Answer from the drawing. Dimensions are ordinates in mm from the lowest x, y and z of the part. A direction names the side the tool comes from. Coordinates: 2 decimals unless noted, no trailing zeros. Write each loop counter-clockwise with the first axis right and the second up, starting at its lowest first coordinate (ties: lowest second). Pieces come first, ordered by that corner, then holes.
(1) Determine the mould class of the marked faces 4, 5 and 6 for opening direction Z: pulls with the +Z half, pulls with the -Z half, needs draft (parallel to the pull), parting line crosses it, or undercut.
(2) Given pin 1 (4 mm diameter, centred on y = 18.5, z = 7.5, fed in from -X); pin 2 (8 mm diameter, centred on x = 6, z = 18, fed in from +Y); pin 3 (3 mm diameter, centred on x = 16, z = 16, fed in from +Y); pin 4 (13 mm diameter, centred on y = 33.5, z = 9, fed in from +X), each flat-ended and moving along its own axis, determine where each tip first touches the part or whether it passes through.
(3) The part is cut by section A-A, the plane z = 10.75. Determine the outline of the cut face in (x, y), and give its area (3 significant figures).
(4) Straight lines are drawn through the part: line 1 along Y through (x, z) = (10.25, 13); line 2 along X through (y, z) = (39, 24.5); line 3 along Y through (x, z) = (14.25, 16.5). For each, find the intervals that lie inside material, in ascending order.
(5) The part is cut by section B-B, the plane y = 30. Determine the outline of the cut face in (x, z), and give its area (3 significant figures).
(6) The part is cut by section D-D, the plane z = 13.75. Determine the outline of the cut face in (x, y).
(7) Which of the six approach directions +Z, -Z, +X, -X, +Y, -Y give full straight-line access (tool end or side, diameter ignored) to the marked faces 1, 2 and 3?
(8) The part is cut by section C-C, the plane x = 10.25. Determine the outline of the cut face in (y, z).
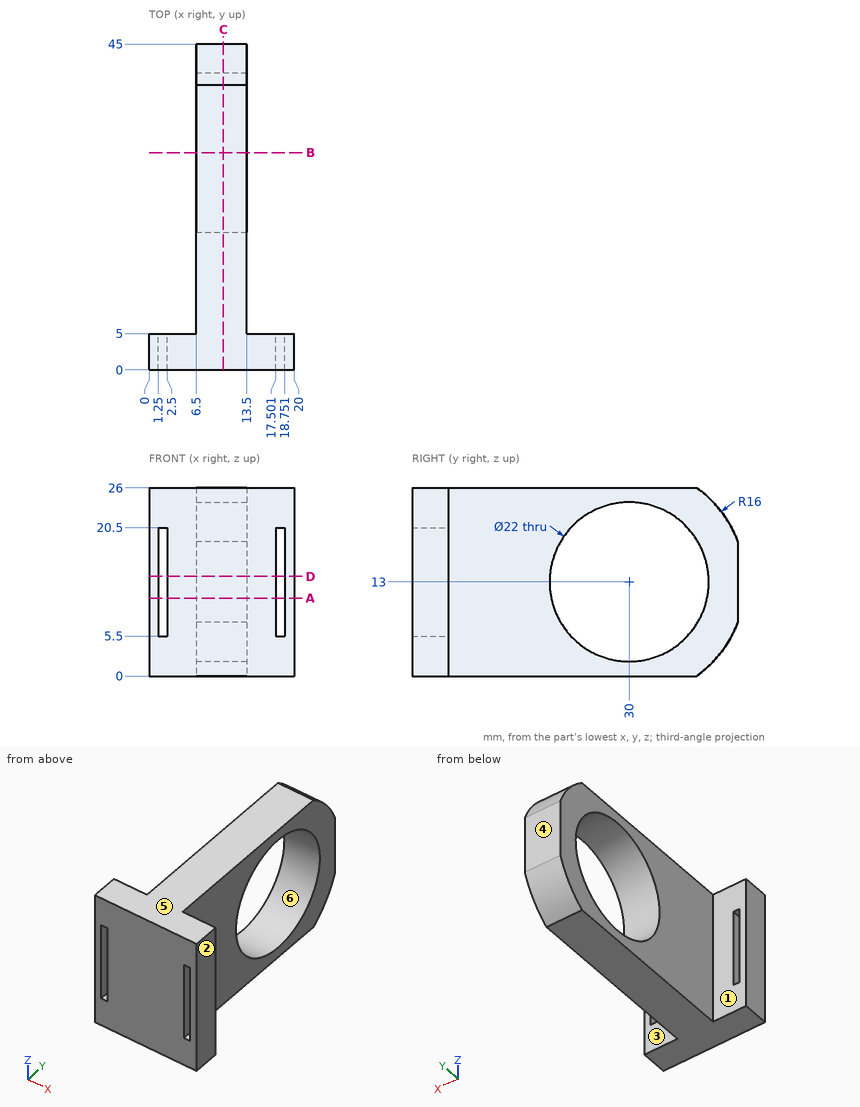
Computed:
1. face 4: needs draft
1. face 5: pulls with the +Z half
1. face 6: undercut
2. pin 1: stops at x = 6.5
2. pin 2: stops at y = 45
2. pin 3: stops at y = 5
2. pin 4: stops at x = 13.5
3. outline: (0, 0) - (1.25, 0) - (1.25, 5) - (0, 5) - close; (2.5, 0) - (17.5, 0) - (17.5, 5) - (13.5, 5) - (13.5, 19.23) - (6.5, 19.23) - (6.5, 5) - (2.5, 5) - close; (6.5, 40.77) - (13.5, 40.77) - (13.5, 45) - (6.5, 45) - close; (18.75, 0) - (20, 0) - (20, 5) - (18.75, 5) - close
3. area: 217 mm2
4. line 1: y = 0 to 19, 41 to 45
4. line 2: x = 6.5 to 13.5
4. line 3: y = 0 to 5
5. outline: (6.5, 0) - (13.5, 0) - (13.5, 2) - (6.5, 2) - close; (6.5, 24) - (13.5, 24) - (13.5, 26) - (6.5, 26) - close
5. area: 28.0 mm2
6. outline: (0, 0) - (1.25, 0) - (1.25, 5) - (0, 5) - close; (2.5, 0) - (17.5, 0) - (17.5, 5) - (13.5, 5) - (13.5, 19.03) - (6.5, 19.03) - (6.5, 5) - (2.5, 5) - close; (6.5, 40.97) - (13.5, 40.97) - (13.5, 45) - (6.5, 45) - close; (18.75, 0) - (20, 0) - (20, 5) - (18.75, 5) - close
7. face 1: +Z, -Z, -X, +Y
7. face 2: +Z, -Z, +X, +Y, -Y
7. face 3: +Z, -Z, +X, +Y
8. outline: (0, 0) - (39.33, 0) arc R16 ccw to (45, 7.43) - (45, 18.57) arc R16 ccw to (39.33, 26) - (0, 26) - close; hole circle Ø22 at (30, 13)
